```python
from build123d import *

# Parameters (mm, degrees)
SKETCH_1_W      = 40
SKETCH_1_H      = 20
EXTRUDE_1_DEPTH = 37.2
SKETCH_2_W      = 54.5
SKETCH_2_H      = 20
SKETCH_2_R      = 1.5
EXTRUDE_2_DEPTH = 3
SKETCH_3_R      = 3
SKETCH_3_R_2    = 1.5
EXTRUDE_3_DEPTH = 6
SKETCH_4_W      = 7.126568636
SKETCH_4_H      = 2.078756753
EXTRUDE_4_DEPTH = 3
EXTRUDE_5_DEPTH = 1


with BuildPart() as part:
    # 草图1 → 凸台-拉伸1 (new body)
    with BuildSketch(Plane(origin=(0, 0, 0), x_dir=(1, 0, 0), z_dir=(0, 1, 0))):
        Rectangle(SKETCH_1_W, SKETCH_1_H)
    extrude(amount=EXTRUDE_1_DEPTH)

    # 草图2 → 凸台-拉伸2 (add)
    with BuildSketch(Plane(origin=(0, 24.5, 0), x_dir=(-1, 0, 0), z_dir=(0, -1, 0))):
        Rectangle(SKETCH_2_W, SKETCH_2_H)
        with Locations(Location((-24.75, 5, 0), (0, 0, 90))):
            Circle(SKETCH_2_R, mode=Mode.SUBTRACT)
        with Locations(Location((-24.75, -5, 0), (0, 0, 90))):
            Circle(SKETCH_2_R, mode=Mode.SUBTRACT)
        with Locations(Location((24.75, -5, 0), (0, 0, 90))):
            Circle(SKETCH_2_R, mode=Mode.SUBTRACT)
        with Locations(Location((24.75, 5, 0), (0, 0, 90))):
            Circle(SKETCH_2_R, mode=Mode.SUBTRACT)
    extrude(amount=-EXTRUDE_2_DEPTH)

    # 草图3 → 凸台-拉伸3 (add)
    with BuildSketch(Plane(origin=(0, 37.2, 0), x_dir=(1, 0, 0), z_dir=(0, 1, 0))):
        with Locations(Location((-11.25, 0, 0), (0, 0, 90))):
            Circle(SKETCH_3_R)
        with Locations(Location((-11.25, 0, 0), (0, 0, 270))):
            Circle(SKETCH_3_R_2, mode=Mode.SUBTRACT)
    extrude(amount=EXTRUDE_3_DEPTH)

    # 草图4 → 凸台-拉伸4 (add)
    with BuildSketch(Plane.ZY.offset(20)):
        with Locations((0, 1.039378376)):
            Rectangle(SKETCH_4_W, SKETCH_4_H)
    extrude(amount=EXTRUDE_4_DEPTH)

    # 草图5 → 凸台-拉伸5 (add, symmetric)
    with BuildSketch(Plane.XY):
        Polygon((-27.25, 27.5), (-20, 30.5), (-20, 27.5), align=None)
        Polygon((20, 27.5), (27.25, 27.5), (20, 30.5), align=None)
    extrude(amount=EXTRUDE_5_DEPTH, both=True)


solid = part.part
```
Geometry: final body of the model. Coordinates: model frame, mm. A direction names the side the tool comes from. Give positions to 0.01 mm unless a question says otherwise; leave off trailing zeros. Loops run counter-clockwise (first coordinate to the right, second up) from the corner with the lowest first, then second, coordinate; pieces in that order, holes last. Notation, with made-up numbers: (-21, 84) -> (-17, 84) arc R19 ccw to (-17, 96) -> close; hole circle Ø11 at (-3.5, 50.5). An arc over 180 degrees is marked (long way). Use one line per item in the form item = value.
Item 1: Section query D-D on x = -11.25. Output: boundary loops of the cut face in (y, z).
A:
outline = (0, -10) -> (37.2, -10) -> (37.2, -3) -> (43.2, -3) -> (43.2, -1.5) -> (37.2, -1.5) -> (37.2, 1.5) -> (43.2, 1.5) -> (43.2, 3) -> (37.2, 3) -> (37.2, 10) -> (0, 10) -> close
Item 2: Pin query (flat end, axial travel): P1, Ø1, axis at y = 0.5, z = -1.5, coming from the -X side; P2, Ø0.9, axis at x = -23.5, y = 29, coming from the -Z side; P3, Ø3.5, axis at x = -24.75, z = -5, coming from the -Y side; P4, Ø0.9, axis at x = 24.5, y = 29.5, coming from the +Z side. Return the tip coordinate at first contact, or that it passes through.
A:
P1 = -23
P2 = -1
P3 = 24.5
P4 = through
Item 3: Section query B-B on z = 0. Output: boundary loops of the cut face in (x, y), and give its area (3 significant figures).
A:
outline = (-27.25, 24.5) -> (-20, 24.5) -> (-20, 2.08) -> (-23, 2.08) -> (-23, 0) -> (20, 0) -> (20, 24.5) -> (27.25, 24.5) -> (27.25, 27.5) -> (20, 30.5) -> (20, 37.2) -> (-8.25, 37.2) -> (-8.25, 43.2) -> (-9.75, 43.2) -> (-9.75, 37.2) -> (-12.75, 37.2) -> (-12.75, 43.2) -> (-14.25, 43.2) -> (-14.25, 37.2) -> (-20, 37.2) -> (-20, 30.5) -> (-27.25, 27.5) -> close
area = 1,580 mm^2
Item 4: Section query C-C on x = -24.75. Output: boundary loops of the cut face in (y, z), and give its area (3 significant figures).
A:
outline = (24.5, -10) -> (27.5, -10) -> (27.5, -6.5) -> (24.5, -6.5) -> close; (24.5, -3.5) -> (27.5, -3.5) -> (27.5, -1) -> (28.53, -1) -> (28.53, 1) -> (27.5, 1) -> (27.5, 3.5) -> (24.5, 3.5) -> close; (24.5, 6.5) -> (27.5, 6.5) -> (27.5, 10) -> (24.5, 10) -> close
area = 44.1 mm^2
Item 5: Access query for faces 4 (the face through (20, 32, 0)), 5 (the face through (20, 12, 0)), 6 (the face through (22, 28, 1)), 7 (the face through (23, 27.5, -6)). Directions: +Z, -Z, +X, -X, +Y, -Y. A direction counts if a zero-diameter tool reaches every point of the face in a straight line with its end or side. Return the directions, or none.
A:
face_4 = +X, +Y
face_5 = +Z, -Z, +X, -Y
face_6 = +Z, +X, +Y
face_7 = -Z, +X, +Y
Item 6: Line query: probe 1 along X at (y, z) = (25.4, 5); probe 2 along Z at (x, y) = (-24, 25); probe 3 along X at (y, z) = (41.05, 0). Output: solid intervals per line, ascending.
A:
probe_1 = -27.25 to -26.25, -23.25 to 23.25, 26.25 to 27.25
probe_2 = -10 to -6.3, -3.7 to 3.7, 6.3 to 10
probe_3 = -14.25 to -12.75, -9.75 to -8.25
Item 7: Section query A-A on z = -5. Output: boundary loops of the cut face in (x, y).
A:
outline = (-27.25, 24.5) -> (-26.25, 24.5) -> (-26.25, 27.5) -> (-27.25, 27.5) -> close; (-23.25, 24.5) -> (-20, 24.5) -> (-20, 0) -> (20, 0) -> (20, 24.5) -> (23.25, 24.5) -> (23.25, 27.5) -> (20, 27.5) -> (20, 37.2) -> (-20, 37.2) -> (-20, 27.5) -> (-23.25, 27.5) -> close; (26.25, 24.5) -> (27.25, 24.5) -> (27.25, 27.5) -> (26.25, 27.5) -> close
Item 8: Draft query along Y for faces 1 (the face through (-20, 12, 0)), 2 (the face through (-27.25, 26, 0)), 3 (the face through (-23, 27.5, -6)). Return one class per face: pulls with the +Y half, pulls with the -Y half, needs draft (parallel to the pull), parting line crosses it, or undercut.
A:
face_1 = undercut
face_2 = needs draft
face_3 = pulls with the +Y half
